Verification items for this drawing (mm, ordinates from the low corner). A direction names the side the tool comes from. Give positions to 0.01 mm unless a question says otherwise; leave off trailing zeros. Loops run counter-clockwise (first coordinate to the right, second up) from the corner with the lowest first, then second, coordinate; pieces in that order, holes last. Notation, with made-up numbers: (53, -6.75) -> (85, -6.75) arc R20 cw to (85, 30.25) -> close; hole circle Ø11 at (16.25, 24). An arc over 180 degrees is marked (long way). Write each question's results on one line, items separated by ' | '. Start each with the question number.
Item 1: Scan lines: line 1 along Y through (x, z) = (3.65, 4); line 2 along Z through (x, y) = (2.6, 6). Record each from-to range of solid material in increasing order.
Item 2: Access from +Z, -Z, +X, -X, +Y, -Y to the whole of each face (thin tool, end or side, straight path). Record for the marked faces 1 and 2.
Item 3: Cross-section at B-B on y = 5. Enter the section's corners in (x, z), then the cut area to 3 significant figures.
Item 4: Gauge pin test, flat ends, axial feed: pin 1 Ø1 at (x, z) = (2, 6) entering from +Y; pin 2 Ø1.9 at (x, y) = (1.5, 10) entering from +Z. Record the tip position at first contact, or that the pin passes through.
Item 5: Cross-section at C-C on z = 5.5. Enter the section's corners in (x, y).
Item 6: Cross-section at A-A on x = 1.6. Enter the section's corners in (y, z).
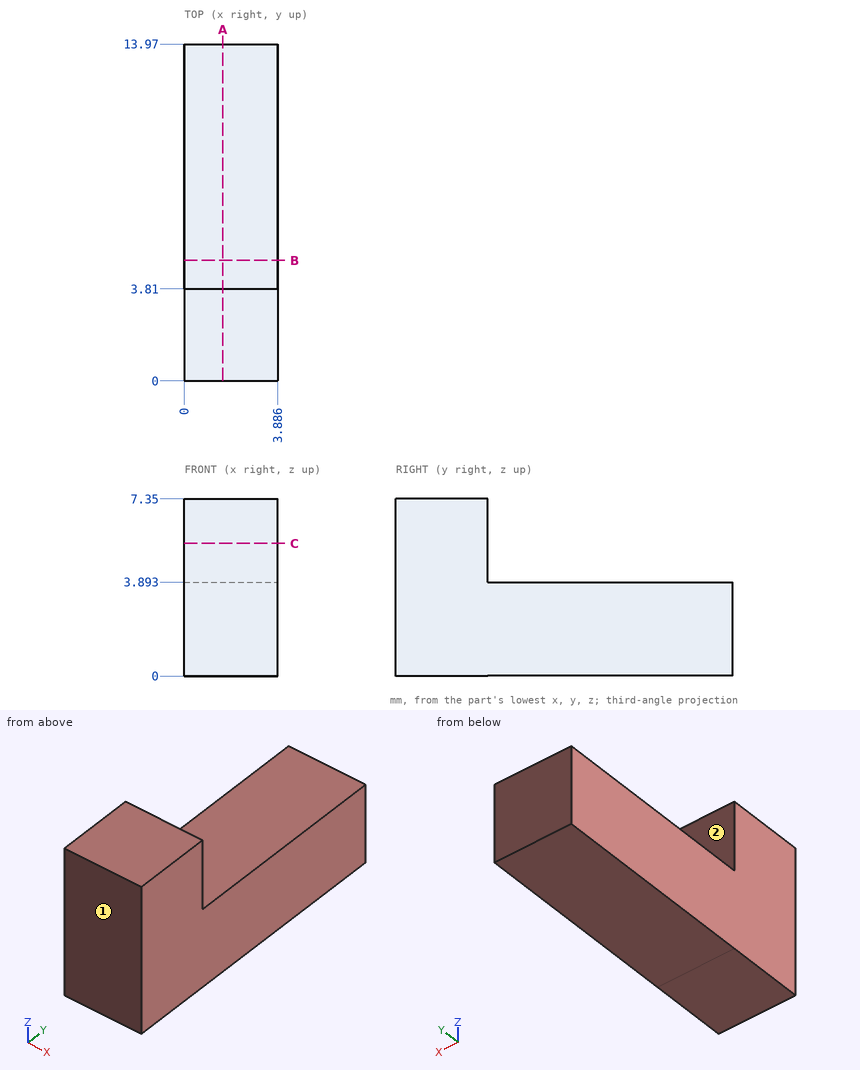
Answer sheet:
1) line 1: y = 0 to 3.81 | line 2: z = 0 to 3.89
2) face 1: +Z, -Z, +X, -X, -Y | face 2: +Z, +X, -X, +Y
3) outline: (0, 0) -> (3.89, 0) -> (3.89, 3.89) -> (0, 3.89) -> close | area: 15.1 mm²
4) pin 1: stops at y = 3.81 | pin 2: stops at z = 3.89
5) outline: (0, 0) -> (3.89, 0) -> (3.89, 3.81) -> (0, 3.81) -> close
6) outline: (0, 0) -> (13.97, 0) -> (13.97, 3.89) -> (3.81, 3.89) -> (3.81, 7.35) -> (0, 7.35) -> close
